```python
from build123d import *

# Parameters (mm, degrees)
SKETCH1_W           = 56.256588963
SKETCH1_H           = 16
SKETCH1_R           = 3.1
SKETCH1_W_2         = 17.2
SKETCH1_H_2         = 3.45
SKETCH1_W_3         = 16
SKETCH1_H_3         = 6.5
BOSS_EXTRUDE1_DEPTH = 3.100997352
SKETCH1_3_R         = 3.1
CUT_EXTRUDE1_DEPTH  = 3.05
SKETCH1_4_W         = 16
SKETCH1_4_H         = 6.5
CUT_EXTRUDE2_DEPTH  = 2.5
SKETCH2_W           = 56.256588963
SKETCH2_H           = 16
SKETCH2_W_2         = 55.856588963
SKETCH2_H_2         = 15.8
CUT_EXTRUDE3_DEPTH  = 3.100997352


with BuildPart() as part:
    # Sketch1 → Boss-Extrude1 (new body)
    # profile 1 of 4: a face of its own
    with BuildSketch(Plane.XY):
        with Locations((-177.370194481, -4)):
            Rectangle(SKETCH1_W, SKETCH1_H)
        with Locations((-153.2419, -5)):
            Circle(SKETCH1_R, mode=Mode.SUBTRACT)
        with Locations((-201.137394481, -5)):
            Circle(SKETCH1_R, mode=Mode.SUBTRACT)
        with Locations((-166.8419, -3.175)):
            Rectangle(SKETCH1_W_2, SKETCH1_H_2, mode=Mode.SUBTRACT)
        with Locations((-186.748488963, -2.799282455)):
            Rectangle(SKETCH1_W_3, SKETCH1_H_3, mode=Mode.SUBTRACT)
    # profile 2 of 4: a face of its own
    with BuildSketch(Plane.XY):
        with Locations((-153.2419, -5)):
            Circle(SKETCH1_R)
    # profile 3 of 4: a face of its own
    with BuildSketch(Plane.XY):
        with Locations((-201.137394481, -5)):
            Circle(SKETCH1_R)
    # profile 4 of 4: a face of its own
    with BuildSketch(Plane.XY):
        with Locations((-186.748488963, -2.799282455)):
            Rectangle(SKETCH1_W_3, SKETCH1_H_3)
    extrude(amount=BOSS_EXTRUDE1_DEPTH)

    # Sketch1<3> → Cut-Extrude1 (cut)
    with BuildSketch(Plane.XY):
        with Locations((-201.137394481, -5)):
            Circle(SKETCH1_3_R)
        with Locations((-153.2419, -5)):
            Circle(SKETCH1_3_R)
    extrude(amount=CUT_EXTRUDE1_DEPTH, mode=Mode.SUBTRACT)

    # Sketch1<4> → Cut-Extrude2 (cut)
    with BuildSketch(Plane.XY):
        with Locations((-186.748488963, -2.799282455)):
            Rectangle(SKETCH1_4_W, SKETCH1_4_H)
    extrude(amount=CUT_EXTRUDE2_DEPTH, mode=Mode.SUBTRACT)

    # Sketch2 → Cut-Extrude3 (cut)
    with BuildSketch(Plane.XY.offset(3.100997352)):
        with Locations((-177.370194481, -4)):
            Rectangle(SKETCH2_W, SKETCH2_H)
        with Locations((-177.370194481, -4)):
            Rectangle(SKETCH2_W_2, SKETCH2_H_2, mode=Mode.SUBTRACT)
    extrude(amount=-CUT_EXTRUDE3_DEPTH, mode=Mode.SUBTRACT)


solid = part.part
```
Verification items for the finished model (mm, model axes). A direction names the side the tool comes from. Round coordinates to 2 decimals unless told otherwise and drop trailing zeros. Write each loop counter-clockwise with the first axis right and the second up, starting at its lowest first coordinate (ties: lowest second). Pieces come first, ordered by that corner, then holes. Notation, with made-up numbers: (82, -10) - (89, -10) arc R22 ccw to (89, 14) - close; hole circle Ø5 at (11.25, -8.5). An arc over 180 degrees is marked (long way). Answer as a JSON object with one key per item and string values. Group by question number.
Q1. Section check B-B, the plane x = -164.5. Enter the section's corners in (y, z), plus the area to 3 significant figures.
Q2. Mould release check, pull along X, two halves, no side actions. Record for faces 4 (the cylindrical face through (-198.18, -4.07, 1.5)), 5 (the flat face through (-149.442, -4, 2)), 6 (the flat face through (-178, -4, 0)): released by +X, released by -X, zero draft, split by the parting line, or undercut.
Q3. Section check C-C, the plane x = -199. Enter the section's corners in (y, z).
Q4. Go/stop test with flat-tipped pins: pin 1 Ø2 at (x, y) = (-167, -4) entering from +Z; pin 2 Ø3 at (x, y) = (-189.5, -2.5) entering from -Z. Record where each tip stops, or that it passes through.
Q5. Thickness scan on line 1 (Y direction, x = -161, z = 1.75); line 2 (Y direction, x = -186.5, z = 0.3); line 3 (Z direction, x = -185.5, y = -4.5). Record the ranges inside material, lowest first.
Q6. Section check A-A, the plane z = 1.4. Enter the section's corners in (x, y), plus the area to 3 significant figures.
Q7. Section check D-D, the plane y = -6.75. Enter the section's corners in (x, z).
Q8. Tool access check on faces 1 (the flat face through (-178, -4, 3.101)), 2 (the cylindrical face through (-150.285, -4.069, 1.504)), 3 (the flat face through (-158.242, -3, 2)). Record the directions out of +Z, -Z, +X, -X, +Y, -Y that give a thin tool (end or side, any length) a straight path to the whole face; none if there is none.
Found:
{
 "1": {"outline": "(-11.9, 0) - (-4.9, 0) - (-4.9, 3.1) - (-11.9, 3.1) - close; (-1.45, 0) - (3.9, 0) - (3.9, 3.1) - (-1.45, 3.1) - close", "area": "38.3 mm^2"},
 "2": {"face 4": "undercut", "face 5": "released by +X", "face 6": "zero draft"},
 "3": {"outline": "(-11.9, 0) - (-7.25, 0) - (-7.25, 3.05) - (-2.75, 3.05) - (-2.75, 0) - (3.9, 0) - (3.9, 3.1) - (-11.9, 3.1) - close"},
 "4": {"pin 1": "stops at z = 3.1", "pin 2": "stops at z = 2.5"},
 "5": {"line 1": "y = -11.9 to -4.9, -1.45 to 3.9", "line 2": "y = -11.9 to -6.05, 0.45 to 3.9", "line 3": "z = 2.5 to 3.1"},
 "6": {"outline": "(-205.3, -11.9) - (-149.44, -11.9) - (-149.44, 3.9) - (-205.3, 3.9) - close; hole circle Ø6.2 at (-201.14, -5); hole (-194.75, -6.05) - (-178.75, -6.05) - (-178.75, 0.45) - (-194.75, 0.45) - close; hole (-175.44, -4.9) - (-158.24, -4.9) - (-158.24, -1.45) - (-175.44, -1.45) - close; hole circle Ø6.2 at (-153.24, -5)", "area": "659 mm^2"},
 "7": {"outline": "(-205.3, 0) - (-203.7, 0) - (-203.7, 3.05) - (-198.58, 3.05) - (-198.58, 0) - (-155.8, 0) - (-155.8, 3.05) - (-150.68, 3.05) - (-150.68, 0) - (-149.44, 0) - (-149.44, 3.1) - (-205.3, 3.1) - close"},
 "8": {"face 1": "+Z, +X, -X, +Y, -Y", "face 2": "-Z", "face 3": "+Z, -Z"}
}
